Geometry: final body of the model. Coordinates: model frame, mm. Face numbers are marked on the shaded views. A direction names the side the tool comes from. Give positions to 0.01 mm unless a question says otherwise; leave off trailing zeros. Write each loop counter-clockwise with the first axis right and the second up, starting at its lowest first coordinate (ties: lowest second). Pieces come first, ordered by that corner, then holes. Notation, with made-up numbers: (21, 20) - (61, 20) arc R23 cw to (61, 38) - close; hole circle Ø5 at (-3.75, 0). An arc over 180 degrees is marked (long way). Use CSV: the item, a comma, the result in double quotes. Start each with the question number.
(1) Draft query along X for the marked faces 1, 2 and 3. Return one class per face: released by +X, released by -X, zero draft, split by the parting line, or undercut.
(2) Section A-A on x = 82. Output: boundary loops of the cut face in (y, z).
(3) Reachability of the marked faces 4, 5, 6, 7 and 8 from +Z, -Z, +X, -X, +Y, -Y: full face, straight path, thin tool, end or side. Return the list, or none.
(4) First-contact query: pin 1 Ø0.6 at (x, z) = (-1, 9.5) entering from +Y; pin 2 Ø2 at (y, z) = (20, 12) entering from -X. Flat tips, straight axial feed; report the tip coordinate or a pass-through.
(5) Section D-D on y = 82. Output: boundary loops of the cut face in (x, z).
(6) Section C-C on z = 3. Output: boundary loops of the cut face in (x, y).
(7) Line query: probe 1 along Y at (x, z) = (2, 28); probe 2 along X at (y, z) = (4, 4); probe 3 along Y at (x, z) = (59, 9). Output: solid intervals per line, ascending. Write a range as [from, to].
(8) Section B-B on y = 2. Output: boundary loops of the cut face in (x, z).
from build123d import *

# Parameters (mm, degrees)
SKETCH_1_W          = 84
SKETCH_1_H          = 93
EXTRUDE_1_DEPTH     = 35
CUT_EXTRUDE_1_REACH = 132.115
SKETCH_2_R          = 1.5
CUT_EXTRUDE_2_REACH = 132.115
SKETCH_3_W          = 58
SKETCH_3_H          = 18
SKETCH_6_W          = 35
SKETCH_6_H          = 10
EXTRUDE_3_DEPTH     = 2


with BuildPart() as part:
    # 草图1 → 凸台-拉伸1 (new body)
    with BuildSketch(Plane.XY):
        with Locations((42, 46.5)):
            Rectangle(SKETCH_1_W, SKETCH_1_H)
    extrude(amount=EXTRUDE_1_DEPTH)

    # 草图2 → 切除-拉伸1 (cut, up to next)
    with BuildSketch(Plane.XY.offset(35), mode=Mode.PRIVATE) as cut_extrude_1_sk1:
        with Locations((82, 2)):
            Circle(SKETCH_2_R)
    cut_extrude_1_tool1 = extrude(cut_extrude_1_sk1.sketch, amount=-CUT_EXTRUDE_1_REACH, mode=Mode.PRIVATE) & part.part
    # 草图2 → 切除-拉伸1 (cut, up to next)
    with BuildSketch(Plane.XY.offset(35), mode=Mode.PRIVATE) as cut_extrude_1_sk2:
        with Locations((2, 2)):
            Circle(SKETCH_2_R)
    cut_extrude_1_tool2 = extrude(cut_extrude_1_sk2.sketch, amount=-CUT_EXTRUDE_1_REACH, mode=Mode.PRIVATE) & part.part
    # 草图2 → 切除-拉伸1 (cut, up to next)
    with BuildSketch(Plane.XY.offset(35), mode=Mode.PRIVATE) as cut_extrude_1_sk3:
        with Locations((82, 82)):
            Circle(SKETCH_2_R)
    cut_extrude_1_tool3 = extrude(cut_extrude_1_sk3.sketch, amount=-CUT_EXTRUDE_1_REACH, mode=Mode.PRIVATE) & part.part
    # 草图2 → 切除-拉伸1 (cut, up to next)
    with BuildSketch(Plane.XY.offset(35), mode=Mode.PRIVATE) as cut_extrude_1_sk4:
        with Locations((2, 82)):
            Circle(SKETCH_2_R)
    cut_extrude_1_tool4 = extrude(cut_extrude_1_sk4.sketch, amount=-CUT_EXTRUDE_1_REACH, mode=Mode.PRIVATE) & part.part
    add(cut_extrude_1_tool1.solids().sort_by_distance((82, 2, 35))[0], mode=Mode.SUBTRACT)
    add(cut_extrude_1_tool2.solids().sort_by_distance((2, 2, 35))[0], mode=Mode.SUBTRACT)
    add(cut_extrude_1_tool3.solids().sort_by_distance((82, 82, 35))[0], mode=Mode.SUBTRACT)
    add(cut_extrude_1_tool4.solids().sort_by_distance((2, 82, 35))[0], mode=Mode.SUBTRACT)

    # 草图3 → 切除-拉伸2 (cut, up to next)
    with BuildSketch(Plane.XY.offset(35), mode=Mode.PRIVATE) as cut_extrude_2_sk1:
        with Locations((42, 9)):
            Rectangle(SKETCH_3_W, SKETCH_3_H)
    cut_extrude_2_tool1 = extrude(cut_extrude_2_sk1.sketch, amount=-CUT_EXTRUDE_2_REACH, mode=Mode.PRIVATE) & part.part
    add(cut_extrude_2_tool1.solids().sort_by_distance((42, 9, 35))[0], mode=Mode.SUBTRACT)

    # 草图6 → 凸台-拉伸3 (add)
    with BuildSketch(Plane(origin=(84, 0, 0), x_dir=(0, 0, -1), z_dir=(1, 0, 0))):
        with Locations((-17.5, 5)):
            Rectangle(SKETCH_6_W, SKETCH_6_H)
    extrude_3 = extrude(amount=EXTRUDE_3_DEPTH)

    # 镜向1: 凸台-拉伸3 across plane
    add(extrude_3.mirror(Plane(origin=(42, 0, 0), x_dir=(0, 0, 1), z_dir=(1, 0, 0))))


solid = part.part
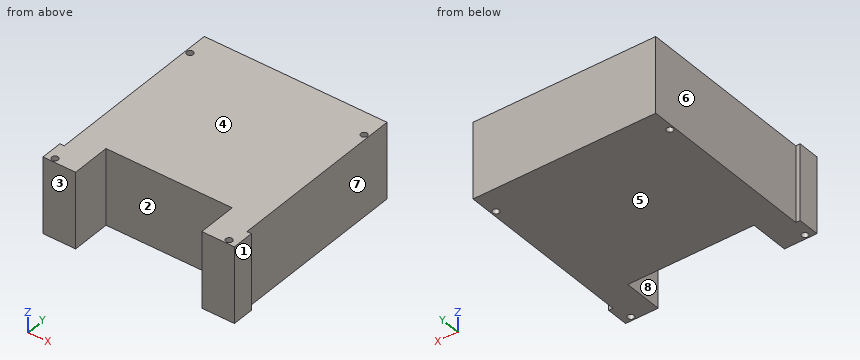
Check values:
1,face 1,"released by +X"
1,face 2,"undercut"
1,face 3,"zero draft"
2,outline,"(0, 0) - (0.5, 0) - (0.5, 35) - (0, 35) - close; (3.5, 0) - (80.5, 0) - (80.5, 35) - (3.5, 35) - close; (83.5, 0) - (93, 0) - (93, 35) - (83.5, 35) - close"
3,face 4,"+Z, +X, -X, +Y, -Y"
3,face 5,"-Z, +X, -X, +Y, -Y"
3,face 6,"+Z, -Z, -X, +Y"
3,face 7,"+Z, -Z, +X, +Y"
3,face 8,"+Z, -Z, -Y"
4,pin 1,"stops at y = 10"
4,pin 2,"stops at x = 0"
5,outline,"(0, 0) - (0.5, 0) - (0.5, 35) - (0, 35) - close; (3.5, 0) - (80.5, 0) - (80.5, 35) - (3.5, 35) - close; (83.5, 0) - (84, 0) - (84, 35) - (83.5, 35) - close"
6,outline,"(-2, 0) - (13, 0) - (13, 18) - (71, 18) - (71, 0) - (86, 0) - (86, 10) - (84, 10) - (84, 93) - (0, 93) - (0, 10) - (-2, 10) - close; hole circle Ø3 at (2, 2); hole circle Ø3 at (2, 82); hole circle Ø3 at (82, 2); hole circle Ø3 at (82, 82)"
7,probe 1,"y = [0, 0.5], [3.5, 80.5], [83.5, 93]"
7,probe 2,"x = [-2, 13], [71, 86]"
7,probe 3,"y = [18, 93]"
8,outline,"(-2, 0) - (0.5, 0) - (0.5, 35) - (-2, 35) - close; (3.5, 0) - (13, 0) - (13, 35) - (3.5, 35) - close; (71, 0) - (80.5, 0) - (80.5, 35) - (71, 35) - close; (83.5, 0) - (86, 0) - (86, 35) - (83.5, 35) - close"
